Autodesk Inventor part; units mm, degrees
ref_plane "YZ Plane" through (0, 0, 0) normal (1, 0, 0) x (0, 1, 0)
ref_plane "XZ Plane" through (0, 0, 0) normal (0, 1, 0) x (-1, 0, 0)
ref_plane "XY Plane" through (0, 0, 0) normal (0, 0, 1) x (1, 0, 0)
sketch "Sketch2" plane through (0, 0, 0) normal (1, 0, 0) x (0, 1, 0)
  arc A0 (10.8439, 6.6106) -> (-12.7, 0) centre (0, 0) ccw
  line L0 (10.8439, 6.6106) -> (38.1, -38.1)
  line L1 (38.1, -38.1) -> (-12.7, -38.1)
  line L2 (-12.7, -38.1) -> (-12.7, 0)
  line L3 (-25.8661, 0) -> (48.761, 0) construction
  dimension "d0" = 12.7
  dimension "d1" = 50.8
  dimension "d2" = 38.1
extrude "Extrusion1" add sketch "Sketch2" along normal mid plane 25.4
sketch "Sketch4" plane through (12.7, 0, 0) normal (1, 0, 0) x (0, 0, -1)
  point P0 (0, 0)
  point P1 (0, 0)
hole "Hole1" at (12.7, 0, 0) direction (-1, 0, 0) diameter 12.7 end through all
sketch "Sketch3" plane through (-12.7, 0, 0) normal (-1, 0, 0) x (0, 0, 1)
  arc A0 (-5.5133, 18.2348) -> (-19.05, 0) centre (0, 0) ccw
  circle A1 centre (0, 0) radius 6.35 construction
  arc A2 (0, -12.7) -> (6.6106, 10.8439) centre (0, 0) ccw
  line L0 (6.6106, 10.8439) -> (-38.1, 38.1)
  line L1 (-38.1, 38.1) -> (-38.1, -12.7) construction
  line L2 (-38.1, -12.7) -> (0, -12.7)
  line L3 (-19.05, 0) -> (-19.05, -12.7)
  dimension "d5" = 38.1
extrude "Extrusion2" cut sketch "Sketch3" against normal blind 6.35
sketch "Sketch5" plane through (12.7, 38.1, -38.1) normal (0, 0, -1) x (-1, 0, 0)
  line L0 (12.7, -60.96) -> (12.7, 10.16) construction
  point P0 (12.7, -38.1)
  point P1 (12.7, -46.0375)
  dimension "d15" = 7.9375
hole "Hole2" at (0, -7.9375, -38.1) direction (0, 0, 1) diameter 3.9624 depth 13.6144 tip angle 118
pattern_linear "Rectangular Pattern1" count 4 spacing 12.7 along (0, 1, 0) of "Hole2"
fillet "Fillet1" radius 3.175 5 edges at (12.7, -3.4331, 12.2272) (12.7, -12.7, -19.05) (12.7, 24.472, -15.7447) (-12.7, 28.1674, -21.8066) (-12.7, -12.7, -28.575)
properties part number "MOUNT,SPRING,ELEVATOR" material "3D Print Material - chopped carbon Nylon12 (preferred)"
Can you work these out from the model? Positions are in its coordinate system, mm. A direction names the side the tool comes from. Round coordinates to 2 decimals unless told otherwise and drop trailing zeros. Write each loop counter-clockwise with the first axis right and the second up, starting at its lowest first coordinate (ties: lowest second). Pieces come first, ordered by that corner, then holes. Notation, with made-up numbers: (3, 6.25) -> (62, 6.25) arc R25 ccw to (62, 25.25) -> close; hole circle Ø5 at (-33, 89). An arc over 180 degrees is marked (long way). One line per question, with ' | ' between items. Start each with the question number.
1) If we mould it in two halves opening along Y, with no side actions, what happens to faces 1 (the conical face through (0.02, 17.12, -23.5)), 2 (the cylindrical face through (-11.795, 27.491, -22.532)), 3 (the cylindrical face through (1.476, -3.655, 12.163)), 4 (the cylindrical face through (-0.6, 6.65, -31.2))? For each: released by +Y, released by -Y, zero draft, split by the parting line, or undercut.
2) On a 3-axis mill with a long thin cutter (end or side, diameter ignored), from which of +Z, -Z, +X, -X, +Y, -Y can I reach the whole of each face in a straight line? I mean faces 5 (the cylindrical face through (3.04, 6.2, 1.38)), 6 (the cylindrical face through (-0.087, 28.183, -31.197)), 7 (the flat face through (-10, -6, -19.05)). Say none if no direction works.
3) Suppose I cut it at A-A on x = 8. Write out the boundary of the cut face in (y, z), then the cut area to 3 significant figures.
4) I need wall thicknesses on line 1 (Y direction, x = 0, z = -28); line 2 (Y direction, x = 0, z = -31.5); line 3 (Y direction, x = 0, z = -34.25). Which ranges of each line are inside material? Lowest first, please. Write a range as [from, to].
5) Suppose I cut it at B-B on x = -7.25. Write out the boundary of the cut face in (y, z), then the cut area to 3 significant figures.
6) I'm going to push flat-ended pins straight in: P1, Ø1.5, axis at x = 7.5, z = 4.5, coming from the -Y side; P2, Ø3, axis at x = 0, y = -7.94, coming from the +Z side; P3, Ø14.5, axis at y = 0, z = 0, coming from the -X side; P4, Ø6.5, axis at x = 0, y = 30.16, coming from the -Z side. Where does each tip first touch, or does it pass through?
Return value:
1) face 1: undercut | face 2: released by +Y | face 3: split by the parting line | face 4: undercut
2) face 5: +X, -X | face 6: -Z | face 7: +Z, -X, -Y
3) outline: (-12.7, -38.1) -> (38.1, -38.1) -> (10.84, 6.61) arc R12.7 ccw to (-12.7, 0) -> close; hole circle Ø12.7 at (0, 0) | area: 1,620 mm2
4) line 1: y = [-12.7, -9.92], [-5.96, 2.78], [6.74, 15.48], [19.44, 28.18] | line 2: y = [-12.7, -9.92], [-5.96, 2.78], [6.74, 15.48], [19.44, 28.18], [32.14, 34.08] | line 3: y = [-12.7, -9.92], [-5.96, 2.78], [6.74, 15.48], [19.44, 28.18], [32.14, 35.75]
5) outline: (-12.7, -38.1) -> (38.1, -38.1) -> (18.23, -5.51) arc R19.05 cw to (0, -19.05) -> (-12.7, -19.05) -> close | area: 978 mm2
6) P1: stops at y = -12.13 | P2: stops at z = 10.95 | P3: stops at x = -6.35 | P4: stops at z = -38.1
